Work out the finished part from the listing and answer in its coordinate system (mm). Round coordinates to 2 decimals unless told otherwise and drop trailing zeros. Write each loop counter-clockwise with the first axis right and the second up, starting at its lowest first coordinate (ties: lowest second). Pieces come first, ordered by that corner, then holes. Notation, with made-up numbers: (57, 31.25) -> (74, 31.25) arc R23 ccw to (74, 67.25) -> close; hole circle Ø5 at (-32, 54). An arc over 180 degrees is marked (long way). Answer as a JSON object with one key per item and string values. Group by question number.
from build123d import *

# Parameters (mm, degrees)
BOSS_EXTRUDE1_DEPTH = 50
SKETCH3_R           = 15
CUT_EXTRUDE2_DEPTH  = 128.299291


with BuildPart() as part:
    # Sketch2 → Boss-Extrude1 (new body)
    with BuildSketch(Plane(origin=(0, 0, 0), x_dir=(1, 0, 0), z_dir=(0, 1, 0))):
        Polygon((0, 0), (0, 40), (110, 0), (110, -30), (0, -30), align=None)
    extrude(amount=BOSS_EXTRUDE1_DEPTH)

    # Sketch3 → Cut-Extrude2 (cut, through all)
    with BuildSketch(Plane(origin=(-12.846715328, 0, -4.671532847), x_dir=(0.341743063, 0, -0.939793423), z_dir=(0.939793423, 0, 0.341743063))):
        with Locations((37.59173694, 25)):
            Circle(SKETCH3_R)
    extrude(amount=CUT_EXTRUDE2_DEPTH, mode=Mode.SUBTRACT)


solid = part.part
1) A cutting plane is placed at B-B on y = 34. Determine the outline of the cut face in (x, z).
2) Straight lines are drawn through the part: L1, parallel to Y at x = 23, z = -26; L2, parallel to Y at x = 72.5, z = -7; L3, parallel to Z at x = 68.5, y = 19.5. For each, find the intervals that lie inside material, in ascending order.
3) A cutting plane is placed at A-A on y = 42. Determine the outline of the cut face in (x, z).
4) Each of these flat-tipped pins is pushed along its axis until it touches: P1, Ø6, axis at x = 89, y = 20, coming from the -Z side; P2, Ø8, axis at x = 35, z = -33, coming from the +Y side; P3, Ø3, axis at x = 59.5, y = 22, coming from the -Z side. Where does it stop, or does it pass through?
Established:
{
 "1": {"outline": "(0, -27.23) -> (110, 12.77) -> (110, 30) -> (0, 30) -> close"},
 "2": {"L1": "y = 0 to 10.97, 39.03 to 50", "L2": "y = 0 to 11.36, 38.64 to 50", "L3": "z = -0.24 to 30"},
 "3": {"outline": "(0, -40) -> (110, 0) -> (110, 30) -> (0, 30) -> close"},
 "4": {"P1": "stops at z = 5.58", "P2": "passes through", "P3": "stops at z = -3.39"}
}
